Model file for the job. Use its own axes, mm. A direction names the side the tool comes from. Round coordinates to 2 decimals unless told otherwise and drop trailing zeros. Order: outer loops, then holes, each group sorted by start corner. A loop starts at its lowest first (then second) coordinate and runs counter-clockwise, first axis right, second up. Notation, with made-up numbers: (20.5, 8) -> (37.5, 8) arc R14 ccw to (37.5, 33) -> close; hole circle Ø4 at (85, -5). An arc over 180 degrees is marked (long way). Use CSV: the item, a comma, the result in double quotes.
```python
from build123d import *

# Parameters (mm, degrees)
SKETCH1_R                      = 12.5
BOSS_EXTRUDE1_DEPTH            = 17.6
SKETCH2_R                      = 6.875
CUT_EXTRUDE1_DEPTH             = 50.8
SKETCH3_R                      = 8
CUT_EXTRUDE3_DEPTH             = 15.6
CUT_EXTRUDE4_DEPTH             = 25.945139807
BOSS_EXTRUDE2_DEPTH            = 17.6
FILLET1_R                      = 2
SKETCH6_W                      = 25
SKETCH6_H                      = 20.775
BOSS_EXTRUDE3_DEPTH            = 20
M4X0_7_TAPPED_HOLE2_AT_2_COUNT = 2
M4X0_7_TAPPED_HOLE2_AT_2_PITCH = 12.206555616
M4X0_7_TAPPED_HOLE1_D          = 3.3
M4X0_7_TAPPED_HOLE1_DEPTH      = 7
M4X0_7_TAPPED_HOLE1_TIP        = 0.991420021
FILLET4_R                      = 1
FILLET6_R                      = 1
FILLET7_R                      = 2


with BuildPart() as part:
    # Sketch1 → Boss-Extrude1 (new body)
    with BuildSketch(Plane(origin=(0, 0, 0), x_dir=(1, 0, 0), z_dir=(0, 1, 0))):
        with Locations(Location((0, 0, 0), (0, 0, 270))):
            Circle(SKETCH1_R)
    extrude(amount=BOSS_EXTRUDE1_DEPTH)

    # Sketch2 → Cut-Extrude1 (cut)
    with BuildSketch(Plane(origin=(0, 17.6, 0), x_dir=(1, 0, 0), z_dir=(0, 1, 0))):
        with Locations(Location((0, 0, 0), (0, 0, 270))):
            Circle(SKETCH2_R)
    extrude(amount=-CUT_EXTRUDE1_DEPTH, mode=Mode.SUBTRACT)

    # Sketch3 → Cut-Extrude3 (cut)
    with BuildSketch(Plane(origin=(0, 17.6, 0), x_dir=(1, 0, 0), z_dir=(0, 1, 0))):
        with Locations(Location((0, 0, 0), (0, 0, 270))):
            Circle(SKETCH3_R)
    extrude(amount=-CUT_EXTRUDE3_DEPTH, mode=Mode.SUBTRACT)

    # Sketch4 → Cut-Extrude4 (cut, through all)
    with BuildSketch(Plane(origin=(0, 17.6, 0), x_dir=(1, 0, 0), z_dir=(0, 1, 0))):
        with BuildLine():
            ThreePointArc((-6.128355545, 5.142300877), (-0.697245942, 7.969557585), (5.142300877, 6.128355545))
            Line((5.142300877, 6.128355545), (8.034845121, 9.575555539))
            ThreePointArc((8.034845121, 9.575555539), (-1.089446784, 12.452433726), (-9.575555539, 8.034845121))
            Line((-9.575555539, 8.034845121), (-6.128355545, 5.142300877))
        make_face()
    extrude(amount=-CUT_EXTRUDE4_DEPTH, mode=Mode.SUBTRACT)

    # Sketch5 → Boss-Extrude2 (add, through all)
    with BuildSketch(Plane(origin=(0, 17.6, 0), x_dir=(1, 0, 0), z_dir=(0, 1, 0))):
        with BuildLine():
            Line((28.663977541, 7.976615292), (19.211771381, 19.085584129))
            Line((19.211771381, 19.085584129), (8.034845121, 9.575555539))
            ThreePointArc((8.034845121, 9.575555539), (12.499926406, 0.042893271), (8.100371818, -9.520187835))
            Line((8.100371818, -9.520187835), (28.663977541, 7.976615292))
        make_face()
    extrude(amount=-BOSS_EXTRUDE2_DEPTH)

    # Fillet1
    fillet1_edges = [part.edges().sort_by_distance(p)[0] for p in [
        (5.142300877, 9.8, -6.128355545),
        (-6.128355545, 9.8, -5.142300877),
    ]]
    fillet(fillet1_edges, radius=FILLET1_R)

    # Sketch6 → Boss-Extrude3 (add)
    with BuildSketch(Plane(origin=(20.563605723, 0, -17.496803127), x_dir=(-0.6480297454391464, 0, -0.7616150267858922), z_dir=(0.7616150267858922, 0, -0.6480297454391464))):
        with Locations((0, 10.3875)):
            Rectangle(SKETCH6_W, SKETCH6_H)
    extrude(amount=BOSS_EXTRUDE3_DEPTH)

    # Sketch9 → M4x0.7 Tapped Hole2 (revolve, cut)
    with BuildSketch(Plane(origin=(21.602614227, 15.3875, -34.793347907), x_dir=(-0.7616150267858922, 0, 0.6480297454391463), z_dir=(0, 1, 0))):
        Polygon((0, 0), (0, 7.991420021), (1.65, 7), (1.65, 0), align=None)
    m4x0_7_tapped_hole2 = revolve(axis=Axis((17.487625343, 15.3875, -39.629603327), (0.6480297454391463, 0, 0.7616150267858921)), mode=Mode.SUBTRACT)

    # M4x0.7 Tapped Hole2 at 2: M4x0.7 Tapped Hole2 ×2
    with Locations(*[Vector(-0.43675753876297707, -0.8192319205190405, 0.3716206570367036) * (i * M4X0_7_TAPPED_HOLE2_AT_2_PITCH) for i in range(1, M4X0_7_TAPPED_HOLE2_AT_2_COUNT)]):
        add(m4x0_7_tapped_hole2, mode=Mode.SUBTRACT)

    # Mirror1: M4x0.7 Tapped Hole2 across plane
    add(m4x0_7_tapped_hole2.mirror(Plane(origin=(0, 0, 0), x_dir=(-0.7616150267858919, 0, 0.6480297454391465), z_dir=(-0.6480297454391465, 0, -0.761615026785892))), mode=Mode.SUBTRACT)

    # Mirror1 copy 1 sketch → Mirror1 copy 1 (revolve, cut)
    with BuildSketch(Plane(origin=(32.472052675, 5.3875, -11.216764019), x_dir=(-0.7616150267858918, 0, 0.6480297454391468), z_dir=(0, 1, 0))):
        Polygon((0, 0), (0, -7.991420021), (1.65, -7), (1.65, 0), align=None)
    revolve(axis=Axis((36.587041559, 5.3875, -6.380508599), (0.6480297454391466, 0, 0.7616150267858917)), mode=Mode.SUBTRACT)

    # M4x0.7 Tapped Hole1
    with Locations(Plane(origin=(0, 17.6, 0), x_dir=(1, 0, 0), z_dir=(0, 1, 0))):
        with Locations((21.749873691, 8.386913416), (12.41680475, 7.010750587)):
            Hole(M4X0_7_TAPPED_HOLE1_D / 2, depth=M4X0_7_TAPPED_HOLE1_DEPTH)
            with Locations((0, 0, -(M4X0_7_TAPPED_HOLE1_DEPTH + M4X0_7_TAPPED_HOLE1_TIP / 2))):  # 118° drill point
                Cone(0, M4X0_7_TAPPED_HOLE1_D / 2, M4X0_7_TAPPED_HOLE1_TIP, mode=Mode.SUBTRACT)

    # Fillet4
    fillet4_edges = [part.edges().sort_by_distance(p)[0] for p in [
        (23.937874461, 17.6, -13.531099711),
    ]]
    fillet(fillet4_edges, radius=FILLET4_R)

    # Fillet6
    fillet6_edges = [part.edges().sort_by_distance(p)[0] for p in [
        (-6.128355545, 1, -5.142300877),
        (5.142300877, 1, -6.128355545),
    ]]
    fillet(fillet6_edges, radius=FILLET6_R)

    # Fillet7
    fillet7_edges = [part.edges().sort_by_distance(p)[0] for p in [
        (19.211771381, 9.3, -19.085584129),
    ]]
    fillet(fillet7_edges, radius=FILLET7_R)


solid = part.part
```
Q1. Probe line 1 along Y through (x, z) = (9, -5.5); line 2 along X through (y, z) = (6.5, 0.5); line 3 along Z through (x, y) = (22.5, 13). List the from-to ranges inside material, lowest first.
From the geometry:
line 1,"y = 0 to 17.6"
line 2,"x = -12.49 to -7.98, 7.98 to 18.7"
line 3,"z = -35.56 to -9.86, -6.92 to -2.73"
Q2. Pin check, flat tips, straight feed: pin 1 (15.5 mm diameter, centred on x = 14, z = -8, fed in from +Y); pin 2 (3 mm diameter, centred on x = -0.5, z = -9, fed in from +Y); pin 3 (10 mm diameter, centred on x = 12, y = 18.5, fed in from +Z). Stop position of each tip, or through.
From the geometry:
pin 1,"stops at y = 17.6"
pin 2,"stops at y = 2"
pin 3,"stops at z = 10.3"
Q3. Cut at B-B (z = 0). Give the cut face in (x, y) (3 decimals).
From the geometry:
outline,"(-12.5, 0) -> (-6.875, 0) -> (-6.875, 2) -> (-8, 2) -> (-8, 17.6) -> (-12.5, 17.6) -> close; (6.875, 0) -> (19.289, 0) -> (19.289, 17.6) -> (8, 17.6) -> (8, 2) -> (6.875, 2) -> close"
Q4. Cut at C-C (y = 12). Give the cut face in (x, z), plus the area to 3 significant figures.
From the geometry:
outline,"(-9.58, -8.03) -> (-7.51, -6.3) arc R2 ccw to (-7.03, -3.81) arc R8 cw (long way) to (6.26, -4.98) arc R2 ccw to (6.3, -7.51) -> (8.03, -9.58) -> (17.69, -17.79) arc R2 cw to (17.92, -20.61) -> (12.46, -27.02) -> (27.7, -39.98) -> (43.9, -20.94) -> (8.1, 9.52) arc R12.5 ccw to start; hole circle Ø3.3 at (12.42, -7.01); hole circle Ø3.3 at (21.75, -8.39)"
area,"945 mm²"
Q5. Mould opens along Z. For faces 1 (the flat face through (9, 17.6, -2)), 2 (the cylindrical face through (-6.83, 9.69, -5.16)), 3 (the cylindrical face through (22.997, 17.901, -14.196)), 4 (the cylindrical face through (5.83, 9.69, -6.27)) say: +Z half, -Z half, draft (parallel to the pull), parting line (faces both ways), or undercut.
From the geometry:
face 1,"draft"
face 2,"undercut"
face 3,"+Z half"
face 4,"undercut"
Q6. Which spindle directions (+Z, -Z, +X, -X, +Y, -Y) get a long thin tool onto all of the face, cutting with end or side? Do faces 5 (the cylindrical face through (14.065, 14.051, -7.083)), 6 (the conical face through (21.556, 5.375, -24.487)), 7 (the flat face through (17.08, 12.84, -21.59)). Say none if no direction does.
From the geometry:
face 5,"+Y"
face 6,"none"
face 7,"-X, +Y"
Q7. Cut at A-A (x = 0). Give the cut face in (y, z) (3 decimals).
From the geometry:
outline,"(0, -8) -> (2, -8) -> (2, -6.875) -> (0, -6.875) -> close; (0, 6.875) -> (2, 6.875) -> (2, 8) -> (17.6, 8) -> (17.6, 12.5) -> (0, 12.5) -> close"
